Autodesk Fusion 360 part; units mm, degrees
sketch "Skizze1" plane through (0, 0, 0) normal (0, 0, 1) x (1, 0, 0)
  circle A0 centre (0, 0) radius 3
  line L0 (2.5981, 1.5) -> (-2.5981, 1.5)
  circle A1 centre (0, 0) radius 2
  line L1 (-2.5981, 1.5) -> (-2.5981, 1)
  line L2 (-2.5981, 1) -> (-2.8284, 1)
  line L3 (-2.5981, 1) -> (2.8284, 1)
  line L4 (3, 0) -> (4.5, 0)
  line L5 (4.5, 0) -> (4.5, 1)
  line L6 (4.5, 1) -> (2.8284, 1)
  line L7 (-3, 0) -> (-4.5, 0)
  line L8 (-4.5, 0) -> (-4.5, 1)
  line L9 (-4.5, 1) -> (-2.8284, 1)
  line L10 (0, -3) -> (0, -4.5)
  line L11 (0, -4.5) -> (4.5, -4.5)
  line L12 (4.5, -4.5) -> (4.5, 0)
  line L13 (-4.5, 0) -> (-4.5, -4.5)
  line L14 (-4.5, -4.5) -> (0, -4.5)
  circle A2 centre (0, 0) radius 1.75
  line L15 (0, 1.75) -> (0, -8.25)
  line L16 (0, -8.25) -> (0, -18.25)
  line L17 (0, -8.25) -> (-4.5, -8.25)
  line L18 (-4.5, -8.25) -> (-4.5, -4.5)
  line L19 (0, -8.25) -> (4.5, -8.25)
  line L20 (4.5, -8.25) -> (4.5, -4.5)
  line L21 (4.5, -8.25) -> (4.4512, -8.25)
  line L22 (4.5, -8.25) -> (-4.5, -8.25)
  line L23 (-4.5, -8.25) -> (-4.5, -18.25)
  line L24 (-4.5, -18.25) -> (4.5, -18.25)
  line L25 (4.5, -18.25) -> (4.5, -8.25)
  line L26 (0, 0) -> (1.5, 0)
  line L27 (1.5, 0) -> (1.5, 1)
  line L28 (1.5, 0) -> (1.5, -18.25)
  line L29 (0, 0) -> (-1.5, 0)
  line L30 (-1.5, 0) -> (-1.5, 1)
  line L31 (-1.5, 0) -> (-1.5, -18.25)
  dimension "d2" = 6
  dimension "d3" = 0.5
  dimension "d4" = 1.5
  dimension "d5" = 1.5
  dimension "d6" = 1.5
  dimension "d7" = 4
  dimension "d8" = 3.5
  dimension "d19" = 10
  dimension "d20" = 10
  dimension "d21" = 9
  dimension "d22" = 10
  dimension "d32" = 1.5
  dimension "d33" = 1.5
extrude "Extrusion2" add sketch "Skizze1" along normal blind 2 contours L0 A1 L3 A2 | A1 L3 A2 L27 L28 | A1 A2 L15 L28 | L0 A1 A2 | L3 A2 L27 | A1 A2 L15 L31 | A2 L27 L28 | A2 L15 L26 L28 | L0 A1 L3 A2 | L0 L3 A2 L15 | L0 A2 L15 | L3 A2 L15 L26 L27 | A1 L3 A2 L30 L31 | A2 L15 L29 L31 | L0 A2 L15 | L0 L3 A2 L15 | L3 A2 L15 L29 L30 | A2 L30 L31 | L3 A2 L30
extrude "Extrusion5" add sketch "Skizze1" along normal blind 3 from surface at 2 contours A0 A1 L3 L28 | A0 L4 L11 L12 L28 | A0 L4 L5 L6 | A0 L10 L11 L15 L28 | A0 A1 L15 L28 | A1 L3 A2 L27 L28 | A0 L10 L14 L15 L31 | A0 A1 L15 L31 | A1 A2 L15 L28 | L11 L15 L19 L22 L28 | L11 L19 L20 L21 L22 L28 | L3 A2 L27 | L14 L15 L17 L22 L31 | A1 A2 L15 L31 | A2 L27 L28 | A2 L15 L26 L28 | L3 A2 L15 L26 L27 | A2 L15 L29 L31 | L3 A2 L15 L29 L30 | L3 A2 L30
extrude "Extrusion6" add sketch "Skizze1" along normal blind 7 from surface at 2 contours L16 L19 L22 L24 L28 | L19 L21 L22 L24 L25 L28 | L16 L17 L22 L24 L31
sketch "Skizze2" plane through (0, -18.25, 0) normal (0, -1, 0) x (1, 0, 0)
  line L0 (-1.5, 2) -> (4.5, 2)
  line L1 (4.5, 9) -> (-1.5, 9)
  circle A0 centre (1.5, 5.5) radius 2.5
  line L2 (4.5, 2) -> (4.5, 9)
  line L3 (-1.5, 9) -> (-1.5, 2)
  dimension "d29" = 5
extrude "Extrusion7" cut sketch "Skizze2" against normal blind 9.5 contours A0
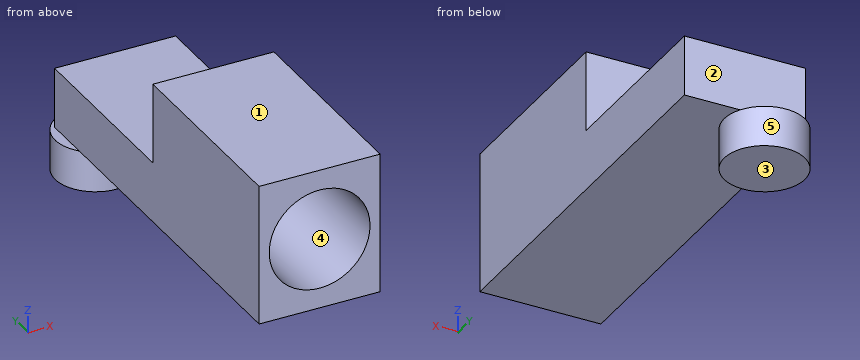
Input: part model. Units: mm. Frame: model coordinates. Face numbers are marked on the shaded views. A direction names the side the tool comes from. Coordinates: 2 decimals unless noted, no trailing zeros. Loops run counter-clockwise (first coordinate to the right, second up) from the corner with the lowest first, then second, coordinate; pieces in that order, holes last.
(1) Section A-A on z = 7. Return the cut outline in (x, y), then the cut area to 3 significant figures.
(2) Section C-C on x = 0. Return the cut outline in (y, z).
(3) Material intervals for probe 1 along Z at (x, y) = (1.5, -11); probe 2 along Y at (x, z) = (3.5, 6.5); probe 3 along X at (y, z) = (-11, 7.5), sorted ascending.
(4) Section B-B on y = -11.75. Return the cut outline in (x, z), then the cut area to 3 significant figures.
(5) Set-up query: the marked faces 1 and 2. Return all of +Z, -Z, +X, -X, +Y, -Y with unobstructed straight access to the full face (end or side cutting, diameter ignored); none if empty.
(6) Section D-D on y = 0. Return the cut outline in (x, z).
(7) Pull-direction query (X, two-part tool) for the marked faces 3, 4 and 5; classes: released by +X, released by -X, zero draft, split by the parting line, or undercut.
(8) First-contact query: pin 1 Ø5 at (y, z) = (-15.5, 3) entering from -X; pin 2 Ø1 at (x, y) = (0, 1) entering from +Z; pin 3 Ø3 at (x, y) = (1, -9.5) entering from -Z; pin 4 Ø2 at (y, z) = (-6.5, 6.5) entering from -X. Flat tips, straight axial feed; report the tip coordinate or a pass-through.
Data:
1. outline: (-1.5, -18.25) - (-0.5, -18.25) - (-0.5, -8.75) - (3.5, -8.75) - (3.5, -18.25) - (4.5, -18.25) - (4.5, -8.25) - (-1.5, -8.25) - close
1. area: 22.0 mm2
2. outline: (-18.25, 2) - (-2, 2) - (-2, 0) - (2, 0) - (2, 2) - (1, 2) - (1, 5) - (-8.25, 5) - (-8.25, 9) - (-18.25, 9) - (-18.25, 7.5) - (-8.75, 7.5) - (-8.75, 3.5) - (-18.25, 3.5) - close
3. probe 1: z = 2 to 3, 8 to 9
3. probe 2: y = -8.75 to -8.25
3. probe 3: x = -1.5 to 0, 3 to 4.5
4. outline: (-1.5, 2) - (4.5, 2) - (4.5, 9) - (-1.5, 9) - close; hole circle Ø5 at (1.5, 5.5)
4. area: 22.4 mm2
5. face 1: +Z, +X, -X, +Y, -Y
5. face 2: +Z, +X, -X, +Y
6. outline: (-2, 0) - (2, 0) - (2, 2) - (4.5, 2) - (4.5, 5) - (-1.5, 5) - (-1.5, 2) - (-2, 2) - close
7. face 3: zero draft
7. face 4: undercut
7. face 5: split by the parting line
8. pin 1: stops at x = -1.5
8. pin 2: stops at z = 5
8. pin 3: stops at z = 2
8. pin 4: passes through
